```python
from build123d import *

# Parameters (mm, degrees)
F1_DEPTH      = 10
F3_R          = 3.5
F4_DEPTH      = 30
F4_DEPTH_BACK = 5


with BuildPart() as f1:
    # F0 (on Top) → F1 (new body)
    with BuildSketch(Plane.XY):
        with BuildLine():
            ThreePointArc((3.3856217223, 7.5), (6.4644660941, 9.3541434669), (10, 10))
            Line((10, 10), (-10, 10))
            Line((-10, 10), (-10, -10))
            Line((-10, -10), (10, -10))
            ThreePointArc((10, -10), (6.4644660941, -9.3541434669), (3.3856217223, -7.5))
            Line((3.3856217223, -7.5), (-7.5, -7.5))
            Line((-7.5, -7.5), (-7.5, 7.5))
            Line((-7.5, 7.5), (3.3856217223, 7.5))
        make_face()
        with BuildLine():
            ThreePointArc((20, 0), (17.0710678119, 7.0710678119), (10, 10))
            Line((10, 10), (10, 7.0710678119))
            ThreePointArc((10, 7.0710678119), (13.623724357, 4.3301270189), (15, 0))
            ThreePointArc((15, 0), (13.623724357, -4.3301270189), (10, -7.0710678119))
            Line((10, -7.0710678119), (10, -10))
            ThreePointArc((10, -10), (17.0710678119, -7.0710678119), (20, 0))
        make_face()
        with BuildLine():
            Line((10, 7.0710678119), (10, 10))
            ThreePointArc((10, 10), (6.4644660941, 9.3541434669), (3.3856217223, 7.5))
            Line((3.3856217223, 7.5), (7.5, 7.5))
            ThreePointArc((7.5, 7.5), (8.7682648404, 7.3919891974), (10, 7.0710678119))
        make_face()
        with BuildLine():
            Line((10, -10), (10, -7.0710678119))
            ThreePointArc((10, -7.0710678119), (8.7682648404, -7.3919891974), (7.5, -7.5))
            Line((7.5, -7.5), (3.3856217223, -7.5))
            ThreePointArc((3.3856217223, -7.5), (6.4644660941, -9.3541434669), (10, -10))
        make_face()
    extrude(amount=F1_DEPTH)


with BuildPart() as f1_1:
    # F2: moved
    add(f1.part.moved(Location((0, 0, -5))))

    # F3 (on face) → F4 (join, two sides)
    with BuildSketch(Plane(origin=(-10, 0, 0), x_dir=(0, -1, 0), z_dir=(-1, 0, 0))) as f4_sk:
        Circle(F3_R)
    extrude(amount=-F4_DEPTH)
    extrude(f4_sk.sketch, amount=F4_DEPTH_BACK)


solid = f1_1.part
```
Input: part model. Units: mm. Frame: model coordinates. A direction names the side the tool comes from. Give positions to 0.01 mm unless a question says otherwise; leave off trailing zeros. Order: outer loops, then holes, each group sorted by start corner. A loop starts at its lowest first (then second) coordinate and runs counter-clockwise, first axis right, second up.
1. Draft query along X for faces 1 (the face through (5, -9, -5)), 2 (the face through (20, 0, 0)), 3 (the face through (-7.5, -1.8, -3.4)). Return one class per face: released by +X, released by -X, zero draft, split by the parting line, or undercut.
Computed:
face 1: zero draft
face 2: released by +X
face 3: undercut
2. Cut plane B-B (x = 11). Return loops of the section in (y, z).
Computed:
outline: (-9.95, -5) - (-6.63, -5) - (-6.63, 5) - (-9.95, 5) - close; circle Ø7 at (0, 0); (6.63, -5) - (9.95, -5) - (9.95, 5) - (6.63, 5) - close
3. Cut plane C-C (z = -2). Return loops of the section in (x, y), and give its area (3 significant figures).
Computed:
outline: (-15, -2.87) - (-10, -2.87) - (-10, -10) - (10, -10) arc R10 ccw to (19.58, -2.87) - (20, -2.87) - (20, 2.87) - (19.58, 2.87) arc R10 ccw to (10, 10) - (-10, 10) - (-10, 2.87) - (-15, 2.87) - close; hole (-7.5, -7.5) - (7.5, -7.5) arc R7.5 ccw to (14.43, -2.87) - (-7.5, -2.87) - close; hole (-7.5, 2.87) - (14.43, 2.87) arc R7.5 ccw to (7.5, 7.5) - (-7.5, 7.5) - close
area: 401 mm2
4. Line query: probe 1 along Y at (x, z) = (5.5, -2.75); probe 2 along Y at (x, z) = (-3.5, 4.5); probe 3 along Y at (x, z) = (5, 2.25). Output: solid intervals per line, ascending.
Computed:
probe 1: y = -10 to -7.5, -2.17 to 2.17, 7.5 to 10
probe 2: y = -10 to -7.5, 7.5 to 10
probe 3: y = -10 to -7.5, -2.68 to 2.68, 7.5 to 10
5. Cut plane A-A (y = 6.25). Return loops of the section in (x, z), and give its area (3 significant figures).
Computed:
outline: (-10, -5) - (-7.5, -5) - (-7.5, 5) - (-10, 5) - close; (11.65, -5) - (17.81, -5) - (17.81, 5) - (11.65, 5) - close
area: 86.6 mm2
6. Cut plane D-D (y = -4.75). Return loops of the section in (x, z).
Computed:
outline: (-10, -5) - (-7.5, -5) - (-7.5, 5) - (-10, 5) - close; (13.3, -5) - (18.8, -5) - (18.8, 5) - (13.3, 5) - close
7. Set-up query: faces 4 (the face through (3.593, -3.233, -1.341)), 5 (the face through (0, 7.5, 0)), 6 (the face through (0, 10, 0)), 7 (the face through (-15, 0, 0)), 8 (the face through (-12.465, -3.233, -1.341)). Return all of +Z, -Z, +X, -X, +Y, -Y with unobstructed straight access to the full face (end or side cutting, diameter ignored); none if empty.
Computed:
face 4: none
face 5: +Z, -Z
face 6: +Z, -Z, +X, -X, +Y
face 7: +Z, -Z, -X, +Y, -Y
face 8: -X
